The model under review builds one solid part; all positions refer to its coordinate system, in mm. Face numbers are marked on the shaded views. A direction names the side the tool comes from. Round coordinates to 2 decimals unless told otherwise and drop trailing zeros. Order: outer loops, then holes, each group sorted by start corner. A loop starts at its lowest first (then second) coordinate and runs counter-clockwise, first axis right, second up. Notation, with made-up numbers: M 39,3 L 98,3 A25 ccw 98,40 Z; hole C 43.5,29 d4. An arc over 180 degrees is marked long. Answer as a JSON object with one key per item and string values. Group by question number.
1. Add section D-D on x = 31. State the section outline as (y, z) points, and give its area (3 significant figures).
2. To check wall thickness, follow probe 1 along Z at (x, y) = (72.25, 44); probe 2 along X at (y, z) = (41.5, 20.25); probe 3 along Z at (x, y) = (62.5, 23.25). State the ranges of each line that lie inside material, in increasing order. Write a range as [from, to].
3. Add section A-A on x = 62.5. State the section outline as (y, z) points.
4. Machinability: for the marked faces 1 and 2, which of the approach directions +Z, -Z, +X, -X, +Y, -Y give a long, thin tool a straight path to every point of the face, cutting with its end or side? Answer none if there is none.
5. Clearance check with a flat-ended pin moving along its axis: P1, Ø3, axis at x = 36.5, z = 6, coming from the +Y side. State where the tip first meets the part, or that it passes through.
6. Add section C-C on z = 20.5. State the section outline as (x, y) points.
7. Add section B-B on y = 44. State the section outline as (x, z) points, and give its area (3 significant figures).
8. Mouldability with a two-part tool opening along X and no side actions: class the marked faces 3, 4, 5 and 6 as released by +X, released by -X, zero draft, split by the parting line, or undercut.
```python
from build123d import *

# Parameters (mm, degrees)
F1_DEPTH = 25
F2_R     = 3
F3_DEPTH = 50.001
F4_R     = 3
F5_DEPTH = 80.001


with BuildPart() as f1:
    # F0 (on Top) → F1 (new body)
    with BuildSketch(Plane.XY):
        Polygon((10, 50), (0, 50), (0, 0), (32, 0), (40, 10), (48, 0), (80, 0), (80, 50), (70, 50), (70, 30), (10, 30), align=None)
    extrude(amount=F1_DEPTH)

    # F2 (on face) → F3 (cut, through all)
    with BuildSketch(Plane.XZ):
        with Locations((17.5, 10)):
            Circle(F2_R)
        with Locations((62.5, 10)):
            Circle(F2_R)
    extrude(amount=-F3_DEPTH, mode=Mode.SUBTRACT)

    # F4 (on face) → F5 (cut, through all)
    with BuildSketch(Plane(origin=(0, 0, 0), x_dir=(0, -1, 0), z_dir=(-1, 0, 0))):
        with Locations((-44, 12.5)):
            Circle(F4_R)
    extrude(amount=-F5_DEPTH, mode=Mode.SUBTRACT)


solid = f1.part
```
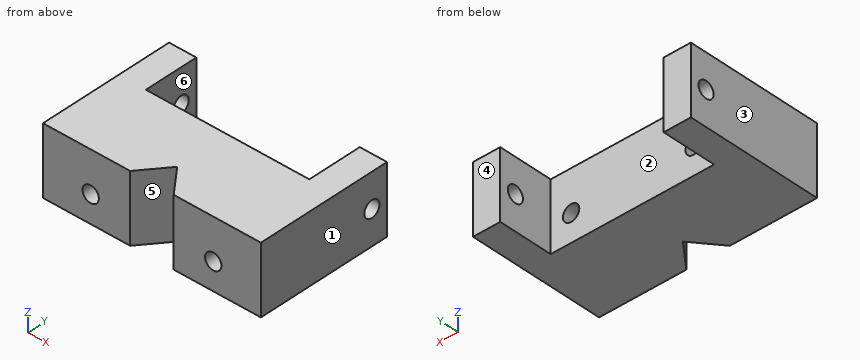
Recorded:
{
 "1": {"outline": "M 0,0 L 30,0 L 30,25 L 0,25 Z", "area": "750 mm²"},
 "2": {"probe 1": "z = [0, 9.5], [15.5, 25]", "probe 2": "x = [0, 10], [70, 80]", "probe 3": "z = [0, 7], [13, 25]"},
 "3": {"outline": "M 0,0 L 30,0 L 30,7 L 0,7 Z; M 0,13 L 30,13 L 30,25 L 0,25 Z"},
 "4": {"face 1": "+Z, -Z, +X, +Y, -Y", "face 2": "+Z, -Z, +Y"},
 "5": {"P1": "stops at y = 30"},
 "6": {"outline": "M 0,0 L 32,0 L 40,10 L 48,0 L 80,0 L 80,50 L 70,50 L 70,30 L 10,30 L 10,50 L 0,50 Z"},
 "7": {"outline": "M 0,0 L 10,0 L 10,9.5 L 0,9.5 Z; M 0,15.5 L 10,15.5 L 10,25 L 0,25 Z; M 70,0 L 80,0 L 80,9.5 L 70,9.5 Z; M 70,15.5 L 80,15.5 L 80,25 L 70,25 Z", "area": "380 mm²"},
 "8": {"face 3": "released by -X", "face 4": "zero draft", "face 5": "undercut", "face 6": "undercut"}
}
